Drawing for the job (mm, zero at the part's lowest x, y, z). Give positions to 0.01 mm unless a question says otherwise; leave off trailing zeros. Write each loop counter-clockwise with the first axis right and the second up, starting at its lowest first coordinate (ties: lowest second). Pieces come first, ordered by that corner, then holes. Notation, with made-up numbers: (-14, 29) - (23, 29) arc R22 ccw to (23, 38) - close; hole circle Ø10 at (28.25, 61.5). An arc over 180 degrees is marked (long way). Write item = value, one per line. Start each with the question number.
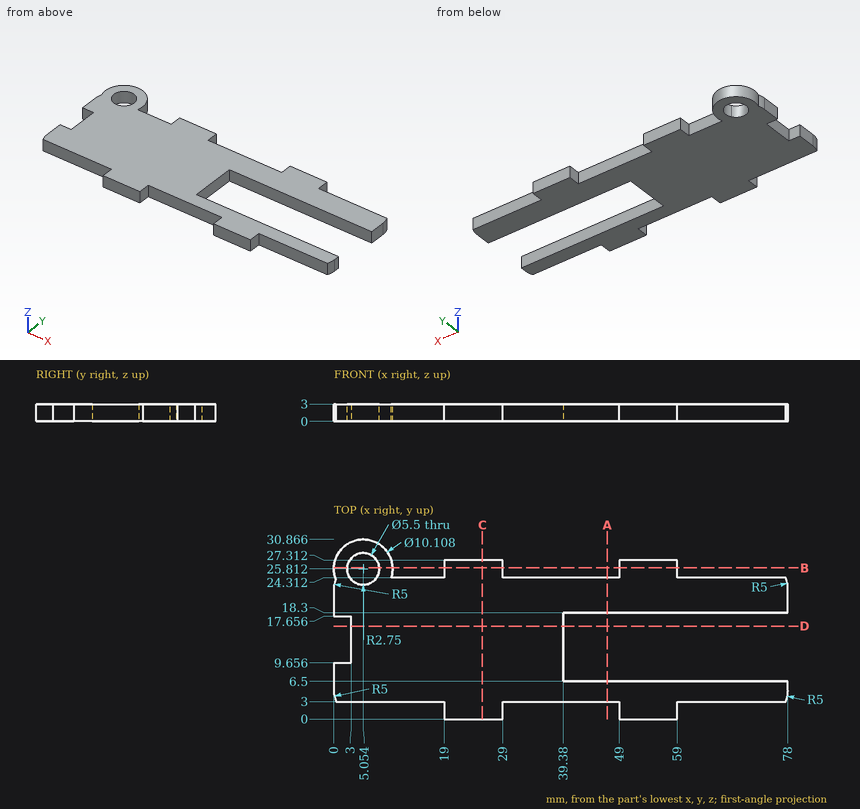
1. Cut at B-B (y = 26). Give the cut face in (x, z) (1 decimal).
2. Pin check, flat tips, straight feed: pin 1 Ø1.5 at (x, z) = (55, 1) entering from -Y; pin 2 Ø1.5 at (x, z) = (5.5, 1.5) entering from -Y; pin 3 Ø1.5 at (y, z) = (1.5, 1) entering from -X; pin 4 Ø1.5 at (x, z) = (15.5, 1.5) entering from +Y. Stop position of each tip, or through.
3. Cut at A-A (x = 47). Give the cut face in (y, z).
4. Cut at D-D (y = 16). Give the cut face in (x, z).
5. Cut at C-C (x = 25.5). Give the cut face in (y, z).
6. Wall check: line 1 along Y through (x, z) = (66.5, 1.45); line 2 along Y through (x, z) = (57, 0.5); line 3 along X through (y, z) = (25.5, 1.95) (1 decimal). Give the ranges that are in metal, low to high.
Output:
q1.outline = (0, 0) - (2.3, 0) - (2.3, 3) - (0, 3) - close; (7.8, 0) - (10.1, 0) - (10.1, 3) - (7.8, 3) - close; (19, 0) - (29, 0) - (29, 3) - (19, 3) - close; (49, 0) - (59, 0) - (59, 3) - (49, 3) - close
q2.pin_1 = 0
q2.pin_2 = 3
q2.pin_3 = 19
q2.pin_4 = 24.31
q3.outline = (3, 0) - (6.5, 0) - (6.5, 3) - (3, 3) - close; (18.3, 0) - (24.31, 0) - (24.31, 3) - (18.3, 3) - close
q4.outline = (3, 0) - (39.38, 0) - (39.38, 3) - (3, 3) - close
q5.outline = (0, 0) - (27.31, 0) - (27.31, 3) - (0, 3) - close
q6.line_1 = 3 to 6.5, 18.3 to 24.31
q6.line_2 = 0 to 6.5, 18.3 to 27.31
q6.line_3 = 0 to 2.3, 7.8 to 10.1, 19 to 29, 49 to 59
